```python
from build123d import *

# Parameters (mm, degrees)
F0_R     = 3.5
F1_DEPTH = 2
F2_R     = 2.5
F3_DEPTH = 2
F4_R     = 1.4
F5_DEPTH = 12
F6_R     = 1


with BuildPart() as f1:
    # F0 (on Top) → F1 (new body)
    with BuildSketch(Plane.XY):
        Circle(F0_R)
    extrude(amount=F1_DEPTH)

    # F2 (on face) → F3 (join)
    with BuildSketch(Plane.XY.offset(2)):
        Circle(F2_R)
    extrude(amount=F3_DEPTH)

    # F4 (on face) → F5 (join)
    with BuildSketch(Plane.XY.offset(4)):
        Circle(F4_R)
    extrude(amount=F5_DEPTH)

    # F6
    f6_edges = [f1.edges().sort_by_distance(p)[0] for p in [
        (-1.4, 0, 16),
    ]]
    fillet(f6_edges, radius=F6_R)


solid = f1.part
```
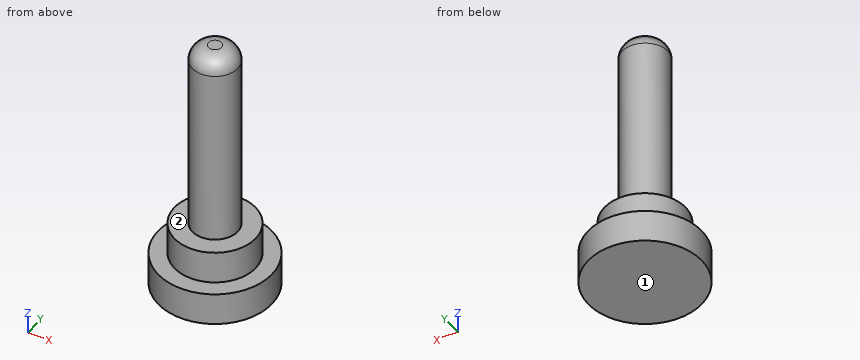
The model under review builds one solid part; all positions refer to its coordinate system, in mm. Face numbers are marked on the shaded views. A direction names the side the tool comes from. Round coordinates to 2 decimals unless told otherwise and drop trailing zeros. Write each loop counter-clockwise with the first axis right and the second up, starting at its lowest first coordinate (ties: lowest second). Pieces come first, ordered by that corner, then holes.
(1) Machinability: for the marked faces 1 and 2, which of the approach directions +Z, -Z, +X, -X, +Y, -Y give a long, thin tool a straight path to every point of the face, cutting with its end or side? Answer none if there is none.
(2) Insertion check: pin 1 (4 mm diameter, centred on x = 1, y = 0.5, fed in from +Z); pin 2 (1 mm diameter, centred on y = -1, z = 8, fed in from -X); pin 3 (1.5 mm diameter, centred on y = 1, z = 11, fed in from +X). Each pin has a flat end and moves straight along its axis. Give the tip position at first contact, or say it passes through.
(3) We need section A-A on x = -2. Give the boundary of the cut face in (y, z).
(4) We need section C-C on x = -2.75. Give the boundary of the cut face in (y, z).
(5) We need section B-B on z = 10.75. Give the boundary of the cut face in (x, y).
(6) Wall thickness on L1, parallel to Y at x = 0, z = 12.5; L2, parallel to Z at x = 2.5, y = -1.5; L3, parallel to Z at x = -0.75, y = 1.75: over which ranges is each line inside the solid? List them lowest first.
Findings below:
1. face 1: -Z, +X, -X, +Y, -Y
1. face 2: +Z
2. pin 1: stops at z = 16
2. pin 2: stops at x = -1.31
2. pin 3: stops at x = 1.38
3. outline: (-2.87, 0) - (2.87, 0) - (2.87, 2) - (1.5, 2) - (1.5, 4) - (-1.5, 4) - (-1.5, 2) - (-2.87, 2) - close
4. outline: (-2.17, 0) - (2.17, 0) - (2.17, 2) - (-2.17, 2) - close
5. outline: circle Ø2.8 at (0, 0)
6. L1: y = -1.4 to 1.4
6. L2: z = 0 to 2
6. L3: z = 0 to 4
